Build history of the part. All positions in model axes, mm. Face numbers are marked on the shaded views. A direction names the side the tool comes from. Give positions to 0.01 mm unless a question says otherwise; leave off trailing zeros. Write each loop counter-clockwise with the first axis right and the second up, starting at its lowest first coordinate (ties: lowest second). Pieces come first, ordered by that corner, then holes. Notation, with made-up numbers: (-30.75, 17) -> (22.25, 17) arc R19 cw to (22.25, 27) -> close; hole circle Ø9 at (9.25, -13.75). An arc over 180 degrees is marked (long way). Put each result on its own line as item: value.
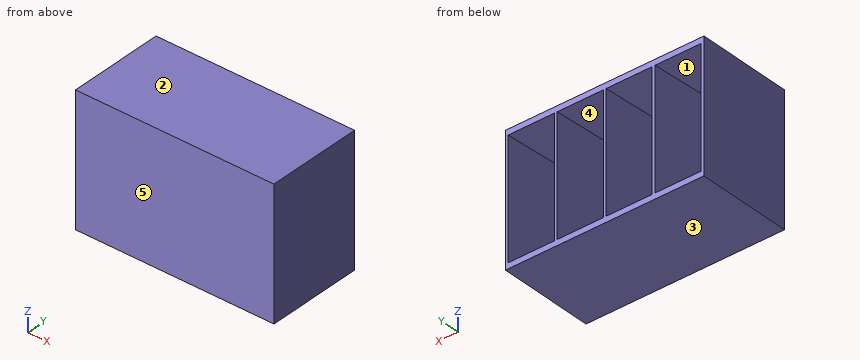
from build123d import *

# Parameters (mm, degrees)
BOSS_EXTRUDE1_DEPTH = 146.05
BOSS_EXTRUDE2_DEPTH = 6.35


with BuildPart() as part:
    # Sketch1 → Boss-Extrude1 (new body)
    with BuildSketch(Plane.XY):
        Polygon((0, 0), (0, 107.95), (3.175, 107.95), (7.6109518, 6.35), (50.7909518, 6.35), (55.226903599, 107.95), (58.401903599, 107.95), (62.837855399, 6.35), (106.017855399, 6.35), (110.453807198, 107.95), (113.628807198, 107.95), (118.064758998, 6.35), (161.244758998, 6.35), (165.680710797, 107.95), (168.855710797, 107.95), (173.291662597, 6.35), (216.471662597, 6.35), (220.907614396, 107.95), (224.082614396, 107.95), (224.082614396, 0), align=None)
    extrude(amount=BOSS_EXTRUDE1_DEPTH)

    # Sketch2 → Boss-Extrude2 (add)
    with BuildSketch(Plane.XY.offset(146.05)):
        Polygon((3.175, 107.95), (55.226903599, 107.95), (50.7909518, 6.35), (7.6109518, 6.35), align=None)
        Polygon((58.401903599, 107.95), (62.837855399, 6.35), (106.017855399, 6.35), (110.453807198, 107.95), align=None)
        Polygon((113.628807198, 107.95), (118.064758998, 6.35), (161.244758998, 6.35), (165.680710797, 107.95), align=None)
        Polygon((168.855710797, 107.95), (173.291662597, 6.35), (216.471662597, 6.35), (220.907614396, 107.95), align=None)
    boss_extrude2 = extrude(amount=-BOSS_EXTRUDE2_DEPTH)

    # Mirror1: Boss-Extrude2 across plane
    add(boss_extrude2.mirror(Plane(origin=(0, 0, 73.025), x_dir=(1, 0, 0), z_dir=(0, 0, -1))))


solid = part.part
1) Wall check: L1, parallel to Z at x = 127, y = 40; L2, parallel to X at y = 89.5, z = 28.5; L3, parallel to X at y = 75, z = 80.5. Give the ranges that are in metal, low to high.
Filled sheet:
L1: 0 to 6.35, 139.7 to 146.05
L2: 0 to 3.98, 54.42 to 59.21, 109.65 to 114.43, 164.88 to 169.66, 220.1 to 224.08
L3: 0 to 4.61, 53.79 to 59.84, 109.02 to 115.07, 164.24 to 170.29, 219.47 to 224.08
2) Slice it at B-B (y = 67). Write the cut outline in (x, z), plus the area to 3 significant figures.
Filled sheet:
outline: (0, 0) -> (224.08, 0) -> (224.08, 146.05) -> (0, 146.05) -> close; hole (4.96, 6.35) -> (53.44, 6.35) -> (53.44, 139.7) -> (4.96, 139.7) -> close; hole (60.19, 6.35) -> (108.67, 6.35) -> (108.67, 139.7) -> (60.19, 139.7) -> close; hole (115.42, 6.35) -> (163.89, 6.35) -> (163.89, 139.7) -> (115.42, 139.7) -> close; hole (170.64, 6.35) -> (219.12, 6.35) -> (219.12, 139.7) -> (170.64, 139.7) -> close
area: 6,870 mm2
3) Slice it at A-A (z = 13.5). Write the cut outline in (x, y) (3 decimals), plus the area to 3 significant figures.
Filled sheet:
outline: (0, 0) -> (224.083, 0) -> (224.083, 107.95) -> (220.908, 107.95) -> (216.472, 6.35) -> (173.292, 6.35) -> (168.856, 107.95) -> (165.681, 107.95) -> (161.245, 6.35) -> (118.065, 6.35) -> (113.629, 107.95) -> (110.454, 107.95) -> (106.018, 6.35) -> (62.838, 6.35) -> (58.402, 107.95) -> (55.227, 107.95) -> (50.791, 6.35) -> (7.611, 6.35) -> (3.175, 107.95) -> (0, 107.95) -> close
area: 4,840 mm2
4) Tool access for the marked faces 4 and 5: list every direction of +Z, -Z, +X, -X, +Y, -Y with a clear straight run to the whole face (end or side of a thin tool).
Filled sheet:
face 4: +Y
face 5: +Z, -Z, +X, -X, -Y
5) Pin check, flat tip, straight feed: pin 1 (3 mm diameter, centred on x = 85, z = 35.5, fed in from +Y). Stop position of the tip, or through.
Filled sheet:
pin 1: y = 6.35
6) Slice it at D-D (y = 11.5). Write the cut outline in (x, z), plus the area to 3 significant figures.
Filled sheet:
outline: (0, 0) -> (224.08, 0) -> (224.08, 146.05) -> (0, 146.05) -> close; hole (7.39, 6.35) -> (51.02, 6.35) -> (51.02, 139.7) -> (7.39, 139.7) -> close; hole (62.61, 6.35) -> (106.24, 6.35) -> (106.24, 139.7) -> (62.61, 139.7) -> close; hole (117.84, 6.35) -> (161.47, 6.35) -> (161.47, 139.7) -> (117.84, 139.7) -> close; hole (173.07, 6.35) -> (216.7, 6.35) -> (216.7, 139.7) -> (173.07, 139.7) -> close
area: 9,460 mm2
7) Slice it at C-C (x = 97.5). Write the cut outline in (y, z).
Filled sheet:
outline: (0, 0) -> (107.95, 0) -> (107.95, 6.35) -> (6.35, 6.35) -> (6.35, 139.7) -> (107.95, 139.7) -> (107.95, 146.05) -> (0, 146.05) -> close
8) Pull direction Z, two halves, no side cores. Call the marked faces 1, 2 and 3: released by +Z, released by -Z, zero draft, split by the parting line, or undercut.
Filled sheet:
face 1: undercut
face 2: released by +Z
face 3: released by -Z
